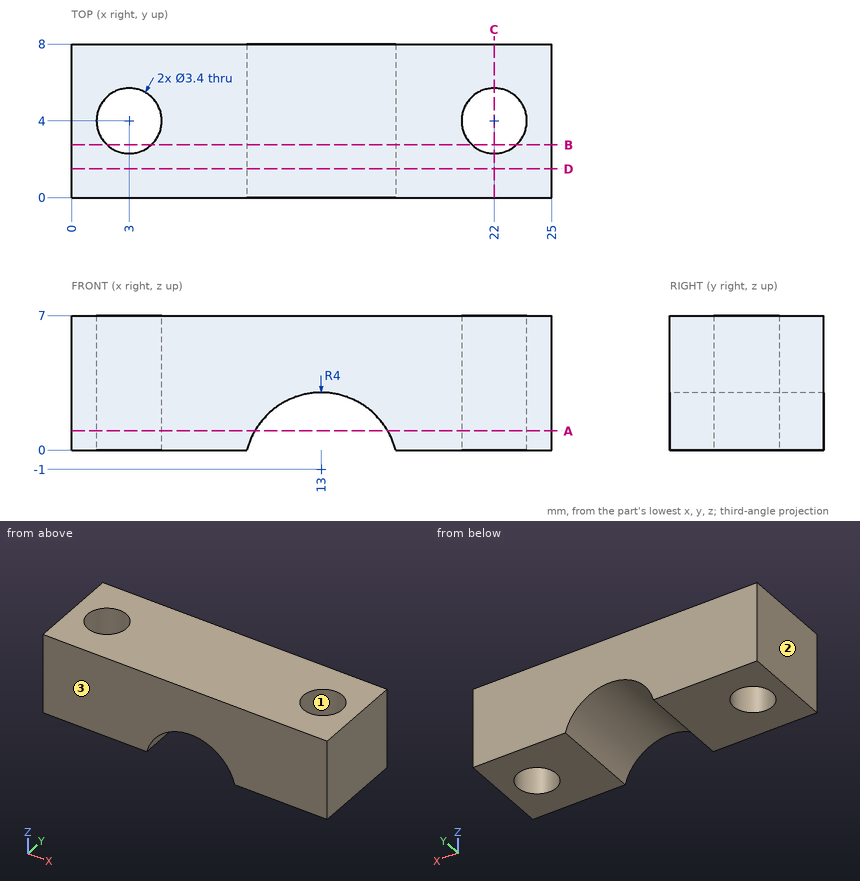
Answer from the drawing. Dimensions are ordinates in mm from the lowest x, y and z of the part. Give positions to 0.01 mm unless a question says otherwise; leave off trailing zeros. Loops run counter-clockwise (first coordinate to the right, second up) from the corner with the lowest first, then second, coordinate; pieces in that order, holes last. Notation, with made-up numbers: (-4.75, 53) -> (32.25, 53) arc R19 cw to (32.25, 75) -> close; hole circle Ø2 at (34.5, 0.5). An arc over 180 degrees is marked (long way). Use a Markdown table: item, result.
Q1. Determine the mould class of the marked faces 1, 2 and 3 for opening direction X: pulls with the +X half, pulls with the -X half, needs draft (parallel to the pull), parting line crosses it, or undercut.
Solved:
| item | result |
|---|---|
| face 1 | undercut |
| face 2 | pulls with the -X half |
| face 3 | needs draft |
Q2. Section A-A, the plane z = 1 is taken. Determine the outline of the cut face in (x, y).
Solved:
| item | result |
|---|---|
| outline | (0, 0) -> (9.54, 0) -> (9.54, 8) -> (0, 8) -> close; (16.46, 0) -> (25, 0) -> (25, 8) -> (16.46, 8) -> close; hole circle Ø3.4 at (3, 4); hole circle Ø3.4 at (22, 4) |
Q3. Find the intervals of material crossed by line 1 along X through (y, z) = (3, 5); line 2 along Y through (x, z) = (3, 1.5); line 3 along X through (y, z) = (7.5, 2.25), in increasing order.
Solved:
| item | result |
|---|---|
| line 1 | x = 0 to 1.63, 4.37 to 20.63, 23.37 to 25 |
| line 2 | y = 0 to 2.3, 5.7 to 8 |
| line 3 | x = 0 to 10.67, 15.33 to 25 |
Q4. Section C-C, the plane x = 22 is taken. Determine the outline of the cut face in (y, z), then the cut area to 3 significant figures.
Solved:
| item | result |
|---|---|
| outline | (0, 0) -> (2.3, 0) -> (2.3, 7) -> (0, 7) -> close; (5.7, 0) -> (8, 0) -> (8, 7) -> (5.7, 7) -> close |
| area | 32.2 mm^2 |
Q5. Section B-B, the plane y = 2.75 is taken. Determine the outline of the cut face in (x, z).
Solved:
| item | result |
|---|---|
| outline | (0, 0) -> (1.85, 0) -> (1.85, 7) -> (0, 7) -> close; (4.15, 0) -> (9.13, 0) arc R4 cw to (16.87, 0) -> (20.85, 0) -> (20.85, 7) -> (4.15, 7) -> close; (23.15, 0) -> (25, 0) -> (25, 7) -> (23.15, 7) -> close |
Q6. Section D-D, the plane y = 1.5 is taken. Determine the outline of the cut face in (x, z), then the cut area to 3 significant figures.
Solved:
| item | result |
|---|---|
| outline | (0, 0) -> (9.13, 0) arc R4 cw to (16.87, 0) -> (25, 0) -> (25, 7) -> (0, 7) -> close |
| area | 158 mm^2 |
